from build123d import *


with BuildPart() as part:
    # Croquis3 → Revolución3 (revolve)
    with BuildSketch(Plane.XY, mode=Mode.PRIVATE) as revoluci_n3_sk:
        with BuildLine():
            Line((0, 0), (90.123101889, 0))
            Line((90.123101889, 0), (97.195601882, 13.872079708))
            ThreePointArc((97.195601882, 13.872079708), (101.267943582, 24.904342215), (102.650891411, 36.582622834))
            Line((102.650891411, 36.582622834), (102.650891411, 55.195630425))
            Line((102.650891411, 55.195630425), (97.650891411, 55.195630425))
            Line((97.650891411, 55.195630425), (97.650891411, 36.582622834))
            ThreePointArc((97.650891411, 36.582622834), (96.406238365, 26.072170277), (92.741130835, 16.143134021))
            Line((92.741130835, 16.143134021), (87.059948421, 5))
            Line((87.059948421, 5), (5, 5))
            Line((5, 5), (5, 55.195630425))
            Line((5, 55.195630425), (4.518270437, 55.677359988))
            Line((4.518270437, 55.677359988), (0.335866273, 55.677359988))
            Line((0.335866273, 55.677359988), (0, 55.195630425))
            Line((0, 55.195630425), (0, 0))
        make_face()
    revolve(revoluci_n3_sk.sketch.rotate(Axis((0, 55.195630425, 0), (0, -1, 0)), 90), axis=Axis((0, 55.195630425, 0), (0, -1, 0)))


solid = part.part
Can you work these out from the model? Positions are in its coordinate system, mm. A direction names the side the tool comes from. Give positions to 0.01 mm unless a question says otherwise; leave off trailing zeros. Order: outer loops, then holes, each group sorted by start corner. A loop starts at its lowest first (then second) coordinate and runs counter-clockwise, first axis right, second up. Notation, with made-up numbers: M -1,-13.5 L 52,-13.5 A27 cw 52,7.5 Z; hole C 37,50.5 d5. An arc over 180 degrees is marked long. Use one line per item in the form item = value.
Item 1: If I drill on line 1 along X through (y, z) = (50.25, 0); line 2 along Z through (x, y) = (2, 32.5); line 3 along Y through (x, z) = (41.5, -53.5), over which ranges is the centre line in solid material (lowest first)? Write a range as [from, to].
Values follow:
line_1 = [-102.65, -97.65], [-5, 5], [97.65, 102.65]
line_2 = [-102.46, -97.44], [-4.58, 4.58], [97.44, 102.46]
line_3 = [0, 5]
Item 2: Thinking about a two-plate mould opening in X: for faces 3 (the cylindrical face through (-30.83, 46.02, 97.91)), 4 (the flat face through (-1, 5, 18)), 5 (the flat face through (38, 55.196, 91)), which applies, pulls with the +X half, pulls with the -X half, needs draft (parallel to the pull), parting line crosses it, or undercut?
Values follow:
face_3 = parting line crosses it
face_4 = undercut
face_5 = needs draft
Item 3: For faces 1 (the flat face through (-1, 0, 1)), 2 (the cylindrical face through (-66, 45.76, -71.97)), which set-ups out of +Z, -Z, +X, -X, +Y, -Y let a thin tool reach every point of the face, with its end or its side?
Values follow:
face_1 = +Z, -Z, +X, -X, -Y
face_2 = +Y
Item 4: If we section it at A-A, the plane y = 51: Write out the boundary of the cut face in (x, z), and give its area (3 significant figures).
Values follow:
outline = C 0,0 d205.3; C 0,0 d10; hole C 0,0 d195.3
area = 3,220 mm^2
Item 5: Will these pins go through, and if not, where does the flat tip stop? pin 1 Ø6 at (y, z) = (44.5, -46.5) entering from -X; pin 2 Ø1.5 at (y, z) = (38.5, 24.5) entering from +X; pin 3 Ø12 at (y, z) = (42, 55) entering from +X.
Values follow:
pin_1 = -92.98
pin_2 = 99.87
pin_3 = 90.2
Item 6: If we section it at B-B, the plane y = 29: Write out the boundary of the cut face in (x, z).
Values follow:
outline = C 0,0 d204.15; C 0,0 d10; hole C 0,0 d194.01
